Geometry check sheet. Reference: the model listing, model coordinates, mm. A direction names the side the tool comes from. Give positions to 0.01 mm unless a question says otherwise; leave off trailing zeros. Order: outer loops, then holes, each group sorted by start corner. A loop starts at its lowest first (then second) coordinate and runs counter-clockwise, first axis right, second up.
```python
from build123d import *

# Parameters (mm, degrees)
SKETCH1_W           = 22.6
SKETCH1_H           = 12.4
BOSS_EXTRUDE1_DEPTH = 23.5
SKETCH3_W           = 5
SKETCH3_H           = 2.4
BOSS_EXTRUDE2_DEPTH = 12.4
CUT_EXTRUDE1_DEPTH  = 26.974843599
BOSS_EXTRUDE3_DEPTH = 4.25
SKETCH6_R           = 2.5
BOSS_EXTRUDE4_DEPTH = 3.3


with BuildPart() as part:
    # Sketch1 → Boss-Extrude1 (new body)
    with BuildSketch(Plane.XY):
        Rectangle(SKETCH1_W, SKETCH1_H)
    extrude(amount=BOSS_EXTRUDE1_DEPTH)

    # Sketch3 → Boss-Extrude2 (add)
    with BuildSketch(Plane.XZ.offset(6.2)):
        with Locations((13.8, 18.05)):
            Rectangle(SKETCH3_W, SKETCH3_H)
        with Locations((-13.8, 18.05)):
            Rectangle(SKETCH3_W, SKETCH3_H)
    extrude(amount=-BOSS_EXTRUDE2_DEPTH)

    # Sketch4 → Cut-Extrude1 (cut, through all)
    with BuildSketch(Plane.XY.offset(19.25)):
        with BuildLine():
            Line((16.3, 0.55), (16.3, -0.55))
            Line((16.3, -0.55), (14.635164654, -0.55))
            ThreePointArc((14.635164654, -0.55), (12.8, 0), (14.635164654, 0.55))
            Line((14.635164654, 0.55), (16.3, 0.55))
        make_face()
        with BuildLine():
            Line((-16.3, 0.55), (-14.635164654, 0.55))
            ThreePointArc((-14.635164654, 0.55), (-12.8, 0), (-14.635164654, -0.55))
            Line((-14.635164654, -0.55), (-16.3, -0.55))
            Line((-16.3, -0.55), (-16.3, 0.55))
        make_face()
    extrude(amount=-CUT_EXTRUDE1_DEPTH, mode=Mode.SUBTRACT)

    # Sketch5 → Boss-Extrude3 (add)
    with BuildSketch(Plane.XY.offset(23.5)):
        with BuildLine():
            ThreePointArc((0.918604651, 1.488757218), (-11.3, 0), (0.918604651, -1.488757218))
            ThreePointArc((0.918604651, -1.488757218), (1.003329596, -1.355013632), (1.151404787, -1.298983275))
            ThreePointArc((1.151404787, -1.298983275), (2.4, 0), (1.151404787, 1.298983275))
            ThreePointArc((1.151404787, 1.298983275), (1.003329596, 1.355013632), (0.918604651, 1.488757218))
        make_face()
    extrude(amount=BOSS_EXTRUDE3_DEPTH)

    # Sketch6 → Boss-Extrude4 (add)
    with BuildSketch(Plane.XY.offset(27.75)):
        with Locations(Location((-5.1, 0, 0), (0, 0, 180))):
            Circle(SKETCH6_R)
    extrude(amount=BOSS_EXTRUDE4_DEPTH)


solid = part.part
```
Q1. Thickness scan on L1, parallel to Y at x = 13.8, z = 17.8; L2, parallel to Z at x = 7, y = 1; L3, parallel to X at y = 0.25, z = 3. Record the ranges inside material, lowest first.
Q2. Gauge pin test, flat ends, axial feed: P1, Ø1.5, axis at x = 15, y = 2.5, coming from the +Z side; P2, Ø2, axis at y = -4, z = 25, coming from the -X side; P3, Ø6, axis at x = 7, y = 2.5, coming from the +Z side; P4, Ø1.2, axis at x = -13.8, y = 0, coming from the -Z side. Record the tip position at first contact, or that the pin passes through.
Q3. Cross-section at C-C, the plane x = -10.5. Record the boundary of the cut face in (y, z), and give its area (3 significant figures).
Q4. Access from +Z, -Z, +X, -X, +Y, -Y to the whole of each face (thin tool, end or side, straight path). Record for faces 1 (the face through (-11.3, 0, 8)), 2 (the face through (2.4, 0, 25.6)), 3 (the face through (-11.3, 0, 21)), 4 (the face through (-3.1, 1.5, 29.4)).
Q5. Cross-section at A-A, the plane x = 13.8. Record the boundary of the cut face in (y, z), and give its area (3 significant figures).
Q6. Cross-section at D-D, the plane x = -6.5. Record the boundary of the cut face in (y, z).
Q7. Cross-section at B-B, the plane z = 18.5. Record the boundary of the cut face in (x, y).
Answers follow:
1. L1: y = -6.2 to -1, 1 to 6.2
1. L2: z = 0 to 23.5
1. L3: x = -11.3 to 11.3
2. P1: stops at z = 19.25
2. P2: stops at x = -10.53
2. P3: stops at z = 23.5
2. P4: passes through
3. outline: (-6.2, 0) - (6.2, 0) - (6.2, 23.5) - (3.05, 23.5) - (3.05, 27.75) - (-3.05, 27.75) - (-3.05, 23.5) - (-6.2, 23.5) - close
3. area: 317 mm2
4. face 1: -Z, -X, +Y, -Y
4. face 2: +Z, +X
4. face 3: +Z, -X, +Y, -Y
4. face 4: +Z
5. outline: (-6.2, 16.85) - (-1, 16.85) - (-1, 19.25) - (-6.2, 19.25) - close; (1, 16.85) - (6.2, 16.85) - (6.2, 19.25) - (1, 19.25) - close
5. area: 25.0 mm2
6. outline: (-6.2, 0) - (6.2, 0) - (6.2, 23.5) - (6.04, 23.5) - (6.04, 27.75) - (2.07, 27.75) - (2.07, 31.05) - (-2.07, 31.05) - (-2.07, 27.75) - (-6.04, 27.75) - (-6.04, 23.5) - (-6.2, 23.5) - close
7. outline: (-16.3, -6.2) - (16.3, -6.2) - (16.3, -0.55) - (14.64, -0.55) arc R1 cw (long way) to (14.64, 0.55) - (16.3, 0.55) - (16.3, 6.2) - (-16.3, 6.2) - (-16.3, 0.55) - (-14.64, 0.55) arc R1 cw (long way) to (-14.64, -0.55) - (-16.3, -0.55) - close
